Can you work these out from the drawing? Everything is in mm from the part's minimum corner. A direction names the side the tool comes from. Coordinates: 2 decimals unless noted, no trailing zeros. Order: outer loops, then holes, each group sorted by start corner. A loop starts at its lowest first (then second) coordinate and runs counter-clockwise, first axis right, second up. Notation, with made-up numbers: (56, -13.75) -> (82, -13.75) arc R25 ccw to (82, 3.25) -> close; hole circle Ø5 at (-15, -3.75). An arc over 180 degrees is marked (long way). Return JSON: item names as keys, results as strings. Group by question number.
1) For the marked faces 1 and 2, which set-ups out of +Z, -Z, +X, -X, +Y, -Y let a thin tool reach every point of the face, with its end or its side?
2) If we section it at A-A, the plane y = 100: Please give me the cut outline in (x, z).
3) If we section it at B-B, the plane z = 225: Please give me the cut outline in (x, y).
4) If we section it at C-C, the plane y = 172.5: Please give me the cut outline in (x, z).
5) If we section it at D-D, the plane x = 144: Please give me the cut outline in (y, z).
6) Thinking about a two-plate mould opening in Z: for the marked faces 3, 4, 5 and 6, which applies, +Z half, -Z half, draft (parallel to the pull), parting line (faces both ways), or undercut?
7) If I drill on probe 1 along Z at (x, y) = (22, 100); probe 2 along X at (y, z) = (45, 103.5), over which ranges is the centre line in solid material (lowest first)? Write a range as from..to.
8) For pin 1 (5 mm diameter, centred on y = 176.5, z = 173, fed in from -X); pin 2 (15.5 mm diameter, centred on y = 28, z = 199.87, fed in from +X); pin 3 (10 mm diameter, centred on x = 191.5, y = 116.5, fed in from +Z); pin 4 (7.5 mm diameter, centred on y = 100, z = 127.87, fed in from +X), each with a flat end and sliding along its axis, tell me the tip position at first contact or that it passes through.
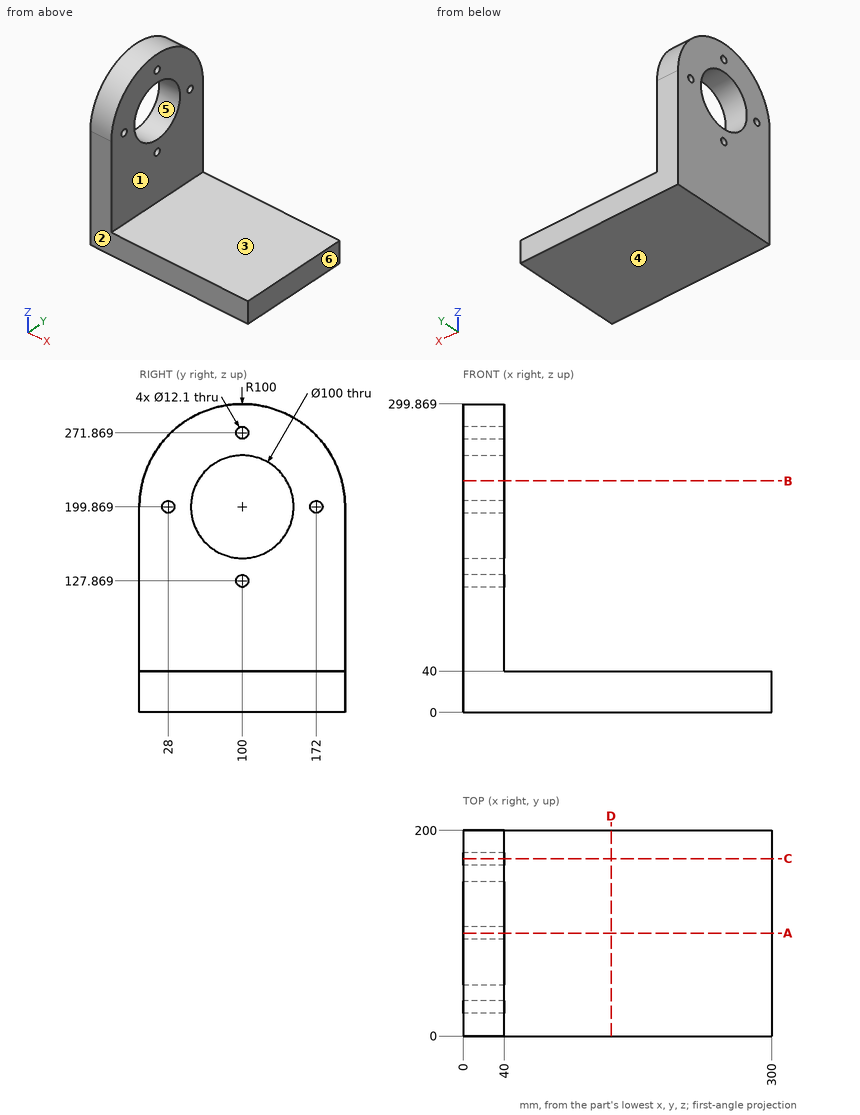
Result sheet:
{
 "1": {"face 1": "+Z, +X, +Y, -Y", "face 2": "+Z, -Z, +X, -X, -Y"},
 "2": {"outline": "(0, 0) -> (300, 0) -> (300, 40) -> (40, 40) -> (40, 121.82) -> (0, 121.82) -> close; (0, 133.92) -> (40, 133.92) -> (40, 149.87) -> (0, 149.87) -> close; (0, 249.87) -> (40, 249.87) -> (40, 265.82) -> (0, 265.82) -> close; (0, 277.92) -> (40, 277.92) -> (40, 299.87) -> (0, 299.87) -> close"},
 "3": {"outline": "(0, 3.21) -> (40, 3.21) -> (40, 56.77) -> (0, 56.77) -> close; (0, 143.23) -> (40, 143.23) -> (40, 196.79) -> (0, 196.79) -> close"},
 "4": {"outline": "(0, 0) -> (300, 0) -> (300, 40) -> (40, 40) -> (40, 193.84) -> (0, 193.84) -> close; (0, 205.9) -> (40, 205.9) -> (40, 268.74) -> (0, 268.74) -> close"},
 "5": {"outline": "(0, 0) -> (200, 0) -> (200, 40) -> (0, 40) -> close"},
 "6": {"face 3": "+Z half", "face 4": "-Z half", "face 5": "undercut", "face 6": "draft"},
 "7": {"probe 1": "z = 0..121.82, 133.92..149.87, 249.87..265.82, 277.92..299.87", "probe 2": "x = 0..40"},
 "8": {"pin 1": "stops at x = 0", "pin 2": "stops at x = 40", "pin 3": "stops at z = 40", "pin 4": "passes through"}
}
